from build123d import *

# Parameters (mm, degrees)
F0_R     = 63.5
F1_DEPTH = 12.7
F2_W     = 25.4
F2_H     = 50.8
F3_DEPTH = 12.7
F2_W_2   = 12.7
F4_DEPTH = 63.5
F6_DEPTH = 88.901
F5_R     = 9.525
F7_DEPTH = 88.901
F8_R     = 3.81


with BuildPart() as f1:
    # F0 (on Top) → F1 (new body)
    with BuildSketch(Plane.XY):
        Circle(F0_R)
        with BuildLine():
            ThreePointArc((-6.33378, 43.996429), (-0.226931, 50.795944), (6.35, 44.45))
            ThreePointArc((6.35, 44.45), (6.345944, 44.223069), (6.33378, 43.996429))
            ThreePointArc((6.33378, 43.996429), (31.430896, 31.430896), (43.996429, 6.33378))
            ThreePointArc((43.996429, 6.33378), (48.776796, 4.647724), (50.8, 0))
            ThreePointArc((50.8, 0), (48.776796, -4.647724), (43.996429, -6.33378))
            ThreePointArc((43.996429, -6.33378), (31.430896, -31.430896), (6.33378, -43.996429))
            ThreePointArc((6.33378, -43.996429), (6.345944, -44.223069), (6.35, -44.45))
            ThreePointArc((6.35, -44.45), (-0.226931, -50.795944), (-6.33378, -43.996429))
            ThreePointArc((-6.33378, -43.996429), (-31.430896, -31.430896), (-43.996429, -6.33378))
            ThreePointArc((-43.996429, -6.33378), (-50.8, 0), (-43.996429, 6.33378))
            ThreePointArc((-43.996429, 6.33378), (-31.430896, 31.430896), (-6.33378, 43.996429))
        make_face(mode=Mode.SUBTRACT)
        with BuildLine():
            ThreePointArc((6.33378, 43.996429), (0, 38.1), (-6.33378, 43.996429))
            ThreePointArc((-6.33378, 43.996429), (-31.430896, 31.430896), (-43.996429, 6.33378))
            ThreePointArc((-43.996429, 6.33378), (-39.802276, 4.326796), (-38.1, 0))
            ThreePointArc((-38.1, 0), (-39.802276, -4.326796), (-43.996429, -6.33378))
            ThreePointArc((-43.996429, -6.33378), (-31.430896, -31.430896), (-6.33378, -43.996429))
            ThreePointArc((-6.33378, -43.996429), (0, -38.1), (6.33378, -43.996429))
            ThreePointArc((6.33378, -43.996429), (31.430896, -31.430896), (43.996429, -6.33378))
            ThreePointArc((43.996429, -6.33378), (38.1, 0), (43.996429, 6.33378))
            ThreePointArc((43.996429, 6.33378), (31.430896, 31.430896), (6.33378, 43.996429))
        make_face()
    extrude(amount=F1_DEPTH)

    # F2 (on face) → F3 (join)
    with BuildSketch(Plane.XY.offset(12.7)):
        Rectangle(F2_W, F2_H)
    extrude(amount=F3_DEPTH)

    # F2 (on face) → F4 (join)
    with BuildSketch(Plane.XY.offset(12.7)):
        with Locations((-19.05, 0)):
            Rectangle(F2_W_2, F2_H)
        with Locations((19.05, 0)):
            Rectangle(F2_W_2, F2_H)
    extrude(amount=F4_DEPTH)

    # F5 (on face) → F6 (cut, through all)
    with BuildSketch(Plane.YZ.offset(25.4)):
        with BuildLine():
            Line((25.4, 76.2), (0, 76.2))
            ThreePointArc((0, 76.2), (17.960512, 68.760512), (25.4, 50.8))
            Line((25.4, 50.8), (25.4, 76.2))
        make_face()
        with BuildLine():
            ThreePointArc((-25.4, 50.8), (-17.960512, 68.760512), (0, 76.2))
            Line((0, 76.2), (-25.4, 76.2))
            Line((-25.4, 76.2), (-25.4, 50.8))
        make_face()
    extrude(amount=-F6_DEPTH, mode=Mode.SUBTRACT)

    # F5 (on face) → F7 (cut, through all)
    with BuildSketch(Plane.YZ.offset(25.4)):
        with Locations((0, 50.8)):
            Circle(F5_R)
    extrude(amount=-F7_DEPTH, mode=Mode.SUBTRACT)

    # F8
    f8_edges = [f1.edges().sort_by_distance(p)[0] for p in [
        (-63.5, 0, 12.7),
        (0, -25.4, 12.7),
        (25.4, 0, 12.7),
        (0, 25.4, 12.7),
        (-25.4, 0, 12.7),
    ]]
    fillet(f8_edges, radius=F8_R)


solid = f1.part
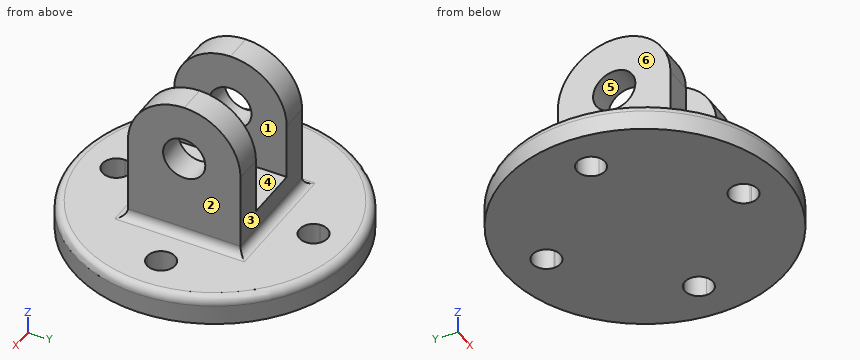
CAD build for the part. Positions are in the model's coordinates, mm. Face numbers are marked on the shaded views. A direction names the side the tool comes from. Round coordinates to 2 decimals unless told otherwise and drop trailing zeros. Order: outer loops, then holes, each group sorted by start corner. A loop starts at its lowest first (then second) coordinate and runs counter-clockwise, first axis right, second up. Notation, with made-up numbers: (-29.5, -20) -> (-23.5, -20) arc R18 cw to (-23.5, -1) -> close; hole circle Ø7 at (-39.75, 46.5). An arc over 180 degrees is marked (long way). Write each question's results on one line, items separated by ' | '.
1. Flat gauge pins, fed straight in: P1, Ø15, axis at y = 4.5, z = 39.5, coming from the +X side; P2, Ø1, axis at x = -4, y = 2.5, coming from the -Z side; P3, Ø12, axis at x = 10.5, z = 47.5, coming from the +Y side; P4, Ø2, axis at x = 25, z = 8.5, coming from the -Y side. Where does each tip first touch, or does it go through?
Findings below:
P1: stops at x = 25.4 | P2: stops at z = 0 | P3: stops at y = 25.4 | P4: stops at y = -58.79
2. Pull direction X, two halves, no side cores. Call the marked faces 4, 5 and 6: pulls with the +X half, pulls with the -X half, needs draft (parallel to the pull), parting line crosses it, or undercut.
Findings below:
face 4: undercut | face 5: needs draft | face 6: pulls with the -X half
3. Cut at A-A (z = 53). Give the cut face in (x, y), plus the area to 3 significant figures.
Findings below:
outline: (-25.4, -25.3) -> (-12.7, -25.3) -> (-12.7, -9.27) -> (-25.4, -9.27) -> close; (-25.4, 9.27) -> (-12.7, 9.27) -> (-12.7, 25.3) -> (-25.4, 25.3) -> close; (12.7, -25.3) -> (25.4, -25.3) -> (25.4, -9.27) -> (12.7, -9.27) -> close; (12.7, 9.27) -> (25.4, 9.27) -> (25.4, 25.3) -> (12.7, 25.3) -> close | area: 815 mm²
4. 3-axis set-ups, long thin cutter, end or side, ignore diameter. For the marked faces 1, 2 and 3: which of +Z, -Z, +X, -X, +Y, -Y reach the whole face in a straight line?
Findings below:
face 1: +Z, +Y, -Y | face 2: +Z, +X, +Y, -Y | face 3: +Z, +X, -X, +Y
5. Wall check: line 1 along Y through (x, z) = (18, 50); line 2 along X through (y, z) = (6, 71); line 3 along Y through (x, z) = (22.5, 16.5). Give the ranges that are in metal, low to high. Write a range as [from, to].
Findings below:
line 1: y = [-25.4, -9.49], [9.49, 25.4] | line 2: x = [-25.4, -12.7], [12.7, 25.4] | line 3: y = [-25.4, 25.4]
